Read the model definition and answer for the solid it produces. Units are mm, in the model's axes. Coordinates: 2 decimals unless noted, no trailing zeros. Loops run counter-clockwise (first coordinate to the right, second up) from the corner with the lowest first, then second, coordinate; pieces in that order, holes last. Notation, with made-up numbers: (42.25, -39.5) -> (81.25, -39.5) arc R8 ccw to (81.25, -27.5) -> close; hole circle Ø11 at (-10, 37). An arc over 180 degrees is marked (long way). One line per question, with ' | ' between items. Start each with the question number.
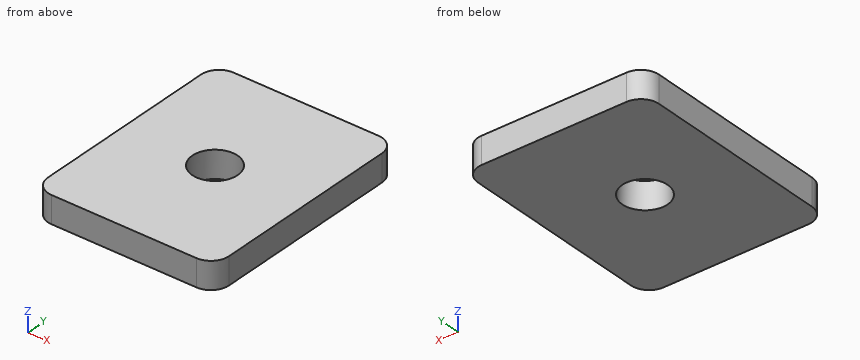
```python
from build123d import *

# Parameters (mm, degrees)
ESQUISSE1_W        = 20
ESQUISSE1_H        = 25
ESQUISSE1_R        = 2.5
BOSS_EXTRU_1_DEPTH = 3
CONG_1_R           = 2


with BuildPart() as part:
    # Esquisse1 → Boss.-Extru.1 (new body)
    with BuildSketch(Plane.XY):
        Rectangle(ESQUISSE1_W, ESQUISSE1_H)
        Circle(ESQUISSE1_R, mode=Mode.SUBTRACT)
    extrude(amount=BOSS_EXTRU_1_DEPTH)

    # Congé1
    cong_1_edges = [part.edges().sort_by_distance(p)[0] for p in [
        (-10, 12.5, 1.5),
        (10, 12.5, 1.5),
        (10, -12.5, 1.5),
        (-10, -12.5, 1.5),
    ]]
    fillet(cong_1_edges, radius=CONG_1_R)


solid = part.part
```
(1) Section C-C on z = 1.05 is taken. Write down the section's boundary in (x, y).
(2) Section B-B on x = 0 is taken. Write down the section's boundary in (y, z), plus the area to 3 significant figures.
(3) Section A-A on y = 0 is taken. Write down the section's boundary in (x, z), plus the area to 3 significant figures.
(4) Each of these flat-tipped pins is pushed along its axis until it touches: pin 1 Ø1 at (x, y) = (-2, -2.5) entering from -Z; pin 2 Ø1 at (x, y) = (0, 0.5) entering from +Z. Where does it stop, or does it pass through?
(5) Find the intervals of material crossed by probe 1 along Y at (x, z) = (0, 1.65); probe 2 along X at (y, z) = (1.25, 0.45); probe 3 along Y at (x, z) = (-1.25, 2.6), in increasing order. Write a range as from..to.
Working result:
1) outline: (-10, -10.5) arc R2 ccw to (-8, -12.5) -> (8, -12.5) arc R2 ccw to (10, -10.5) -> (10, 10.5) arc R2 ccw to (8, 12.5) -> (-8, 12.5) arc R2 ccw to (-10, 10.5) -> close; hole circle Ø5 at (0, 0)
2) outline: (-12.5, 0) -> (-2.5, 0) -> (-2.5, 3) -> (-12.5, 3) -> close; (2.5, 0) -> (12.5, 0) -> (12.5, 3) -> (2.5, 3) -> close | area: 60.0 mm2
3) outline: (-10, 0) -> (-2.5, 0) -> (-2.5, 3) -> (-10, 3) -> close; (2.5, 0) -> (10, 0) -> (10, 3) -> (2.5, 3) -> close | area: 45.0 mm2
4) pin 1: stops at z = 0 | pin 2: passes through
5) probe 1: y = -12.5..-2.5, 2.5..12.5 | probe 2: x = -10..-2.17, 2.17..10 | probe 3: y = -12.5..-2.17, 2.17..12.5
